Autodesk Inventor part; units mm, degrees
ref_plane "YZ Plane" through (0, 0, 0) normal (1, 0, 0) x (0, 1, 0)
ref_plane "XZ Plane" through (0, 0, 0) normal (0, 1, 0) x (-1, 0, 0)
ref_plane "XY Plane" through (0, 0, 0) normal (0, 0, 1) x (1, 0, 0)
sketch "스케치1" plane through (0, 0, 0) normal (0, 0, 1) x (1, 0, 0)
  line L0 (118.1968, 6) -> (118.1968, 0)
  line L1 (0, 0) -> (2.3, 0)
  line L2 (2.3, 0) -> (2.3, -6)
  line L3 (150, -6) -> (2.3, -6)
  line L4 (150, -6) -> (150, 6)
  line L5 (0, 6) -> (150, 6)
  line L6 (0, 0) -> (0, 6)
  line L7 (150, -6) -> (0, -6)
  line L8 (0, -6) -> (0, 0)
  line L9 (0, 0) -> (150, 0)
  line L10 (150, 0) -> (150, -6)
  line L11 (150, -6) -> (144, -6)
  line L12 (144, -6) -> (144, 0)
  line L13 (144, 0) -> (150, 0)
  line L14 (150, 0) -> (150, -6)
  line L15 (122.25, 6) -> (131.75, 6)
  line L16 (128.025, 6) -> (128.025, 0)
  line L17 (125.975, 6) -> (125.975, 0)
  line L18 (127, 0) -> (127, 6)
  line L19 (104, 0) -> (104, -6)
  line L20 (104, -6) -> (110, -6)
  line L21 (110, -6) -> (110, 0)
  line L22 (110, 0) -> (104, 0)
  line L23 (104, 0) -> (104, -6)
  line L24 (75, -6) -> (75, 6)
  line L25 (0, 0) -> (0, -6)
  line L26 (0, -6) -> (6, -6)
  line L27 (6, 0) -> (0, 0)
  line L28 (0, 0) -> (0, -6)
  line L29 (40, 0) -> (46, 0)
  line L30 (150, -6) -> (144, -6)
  line L31 (144, -6) -> (144, 0)
  line L32 (144, 0) -> (150, 0)
  line L33 (150, 0) -> (150, -6)
  line L34 (110, -6) -> (104, -6)
  line L35 (104, -6) -> (104, 0)
  line L36 (104, 0) -> (110, 0)
  line L37 (110, 0) -> (110, -6)
  line L38 (0, 0) -> (0, -6)
  line L39 (0, -6) -> (6, -6)
  line L40 (6, -6) -> (6, 0)
  line L41 (6, 0) -> (0, 0)
  line L42 (0, 0) -> (0, -6)
  line L43 (40, -6) -> (40, 0)
  line L44 (46, -6) -> (40, -6)
  line L45 (46, 0) -> (46, -6)
  line L46 (46, 0) -> (46, -6)
  line L47 (40, 0) -> (46, 0)
  line L48 (0, -6) -> (6, -6)
  line L49 (6, -6) -> (6, 0)
  line L50 (6, 0) -> (0, 0)
  line L51 (0, 0) -> (0, -6)
  line L52 (40, -6) -> (46, -6)
  line L53 (46, -6) -> (46, 0)
  line L54 (46, 0) -> (40, 0)
  line L55 (40, 0) -> (40, -6)
  line L56 (150, 0) -> (0, 0)
  line L57 (0, 0) -> (0, -125.2)
  line L58 (0, -125.2) -> (150, -125.2)
  line L59 (150, -125.2) -> (150, 0)
  line L60 (150, -62.6) -> (0, -62.6)
  line L61 (0, -125.2) -> (2.3, -125.2)
  line L62 (2.3, -125.2) -> (2.3, -119.2)
  line L63 (150, -119.2) -> (2.3, -119.2)
  line L64 (150, -119.2) -> (0, -119.2)
  line L65 (0, -119.2) -> (0, -125.2)
  line L66 (0, -125.2) -> (150, -125.2)
  line L67 (150, -125.2) -> (150, -119.2)
  line L68 (150, -119.2) -> (144, -119.2)
  line L69 (144, -119.2) -> (144, -125.2)
  line L70 (144, -125.2) -> (150, -125.2)
  line L71 (150, -125.2) -> (150, -119.2)
  line L72 (110, -119.2) -> (110, -125.2)
  line L73 (104, -119.2) -> (110, -119.2)
  line L74 (104, -125.2) -> (104, -119.2)
  line L75 (104, -125.2) -> (104, -119.2)
  line L76 (110, -125.2) -> (104, -125.2)
  line L77 (40, -125.2) -> (46, -125.2)
  line L78 (0, -125.2) -> (0, -119.2)
  line L79 (0, -119.2) -> (6, -119.2)
  line L80 (0, -125.2) -> (0, -119.2)
  line L81 (6, -125.2) -> (0, -125.2)
  line L82 (150, -119.2) -> (144, -119.2)
  line L83 (144, -119.2) -> (144, -125.2)
  line L84 (144, -125.2) -> (150, -125.2)
  line L85 (150, -125.2) -> (150, -119.2)
  line L86 (110, -119.2) -> (104, -119.2)
  line L87 (104, -119.2) -> (104, -125.2)
  line L88 (104, -125.2) -> (110, -125.2)
  line L89 (110, -125.2) -> (110, -119.2)
  line L90 (0, -125.2) -> (0, -119.2)
  line L91 (0, -119.2) -> (6, -119.2)
  line L92 (6, -119.2) -> (6, -125.2)
  line L93 (6, -125.2) -> (0, -125.2)
  line L94 (0, -125.2) -> (0, -119.2)
  line L95 (6, -119.2) -> (6, -125.2)
  line L96 (0, -125.2) -> (0, -119.2)
  line L97 (0, -119.2) -> (6, -119.2)
  line L98 (6, -125.2) -> (0, -125.2)
  line L99 (40, -119.2) -> (40, -125.2)
  line L100 (40, -125.2) -> (40, -119.2)
  line L101 (46, -119.2) -> (40, -119.2)
  line L102 (46, -125.2) -> (46, -119.2)
  line L103 (46, -125.2) -> (46, -119.2)
  line L104 (46, -119.2) -> (46, -125.2)
  line L105 (40, -119.2) -> (46, -119.2)
  line L106 (46, -125.2) -> (40, -125.2)
  line L107 (40, -125.2) -> (46, -125.2)
  line L108 (150, -125.2) -> (0, -125.2)
  point P0 (21.975, 0)
  point P1 (24.025, 0)
  point P2 (31.8032, 0)
  point P3 (21.975, 0)
  point P4 (24.025, 0)
  point P5 (23, 0)
  point P6 (118.1968, -125.2)
  point P7 (128.025, -125.2)
  point P8 (125.975, -125.2)
  point P9 (127, -125.2)
  point P10 (75, -119.2)
  point P11 (24.025, -125.2)
  point P12 (21.975, -125.2)
  point P13 (24.025, -125.2)
  point P14 (23, -125.2)
  point P15 (21.975, -125.2)
  point P16 (31.8032, -125.2)
  dimension "d0" = 125.2
extrude "돌출1" add sketch "스케치1" along normal blind 6 contours L9 L12 L3 L21 | L24 L3 L45 L9 | L9 L19 L3 L24 | L3 L59 L60 L57 L7 | L43 L3 L40 L9 | L60 L59 L63 L64 L57
sketch "스케치2" plane through (0, 0, 0) normal (0, 0, -1) x (-1, 0, 0)
  circle A0 centre (-72.2193, -29.1573) radius 1.55
  circle A1 centre (-75, -39.8) radius 1.5
  circle A2 centre (-75, -39.8) radius 13.9
  circle A3 centre (-75, -39.8) radius 5.2
  circle A4 centre (-75, -39.8) radius 1.6
  point P0 (0, 0)
  dimension "d5" = 0.1
extrude "돌출2" cut sketch "스케치2" against normal up to next contours A1 | A4
sketch "스케치5" plane through (0, 0, 6) normal (0, 0, 1) x (1, 0, 0)
  line L0 (6, 0) -> (6, -6)
  line L1 (6, -6) -> (0, -6)
  line L2 (0, -6) -> (0, -119.2)
  line L3 (150, -119.2) -> (150, -6)
  line L4 (150, -6) -> (144, -6)
  line L5 (144, -6) -> (144, 0)
  line L6 (144, 0) -> (110, 0)
  line L7 (110, 0) -> (110, -6)
  line L8 (110, -6) -> (104, -6)
  line L9 (104, -6) -> (104, 0)
  line L10 (104, 0) -> (46, 0)
  line L11 (46, 0) -> (46, -6)
  line L12 (46, -6) -> (40, -6)
  line L13 (40, -6) -> (40, 0)
  line L14 (40, 0) -> (6, 0)
  circle A0 centre (75, -39.8) radius 1.6
  circle A1 centre (40, -6) radius 1
  circle A2 centre (46, -6) radius 1
  circle A3 centre (40, 0) radius 1
  circle A4 centre (46, 0) radius 1
  circle A5 centre (6, 0) radius 1
  line L15 (6, 0) -> (6, -6)
  circle A6 centre (6, -6) radius 1
  circle A7 centre (0, -6) radius 1
  circle A8 centre (104, -6) radius 1
  circle A9 centre (104, 0) radius 1
  line L16 (110, -6) -> (104, -6)
  circle A10 centre (110, -6) radius 1
  circle A11 centre (110, 0) radius 1
  circle A12 centre (144, -6) radius 1
  line L17 (144, 0) -> (110, 0)
  circle A13 centre (144, 0) radius 1
  circle A14 centre (150, -6) radius 1
  circle A15 centre (123.8, -69.5) radius 1
  circle A16 centre (123.8, -63.1) radius 1
  circle A17 centre (130.2, -69.5) radius 1
  line L18 (130.2, -69.5) -> (130.2, -63.1)
  circle A18 centre (130.2, -63.1) radius 1
  circle A19 centre (19.8, -69.5) radius 1
  circle A20 centre (19.8, -63.1) radius 1
  circle A21 centre (26.2, -69.5) radius 1
  circle A22 centre (26.2, -63.1) radius 1
  line L19 (0, -119.2) -> (150, -119.2)
  point P0 (0, 0)
  point P1 (149, -6)
  point P2 (150, -7)
  point P3 (144, -5)
  point P4 (145, -6)
  point P5 (143, 0)
  point P6 (144, -1)
  dimension "d32" = 2
  dimension "d33" = 2
  dimension "d34" = 2
  dimension "d35" = 2
  dimension "d36" = 2
  dimension "d37" = 2
  dimension "d38" = 2
  dimension "d39" = 2
  dimension "d40" = 2
  dimension "d41" = 2
  dimension "d42" = 2
  dimension "d43" = 2
  dimension "d44" = 2
  dimension "d45" = 2
  dimension "d46" = 2
  dimension "d47" = 2
  dimension "d48" = 2
  dimension "d49" = 2
  dimension "d50" = 2
  dimension "d51" = 2
  dimension "d52" = 2
  dimension "d53" = 2
extrude "돌출5" cut sketch "스케치5" against normal up to next contours L14 A5 L0 | L0 A5 L14 | A6 L1 L0 | L0 L1 A6 | A3 L13 L14 | L14 L13 A3 | A7 L2 L1 | L1 L2 A7 | A1 L12 L13 | L13 L12 A1 | A2 L11 L12 | L12 L11 A2 | A14 L4 L3 | A4 L10 L11 | L11 L10 A4 | A12 L5 L4 | A9 L9 L10 | L10 L9 A9 | A13 L6 L5 | A8 L8 L9 | L9 L8 A8 | A11 L7 L6 | L6 L7 A11 | A10 L7 L8 | L8 L7 A10 picked at (149.7812, -6.6253) picked at (143.8112, -6.634) picked at (143.7812, -0.6253)
sketch "스케치6" plane through (0, 0, 6) normal (0, 0, 1) x (1, 0, 0)
  line L0 (6, -6) -> (6, 0)
  line L1 (0, 0) -> (6, 0)
  line L2 (0, -6) -> (0, 0)
  line L3 (0, -6) -> (6, -6)
  line L4 (40, 0) -> (40, -6)
  line L5 (40, -6) -> (46, -6)
  line L6 (46, -6) -> (46, 0)
  line L7 (40, 0) -> (46, 0)
  line L8 (40, 0) -> (6, 0)
  line L9 (23, 0) -> (23, -6)
  circle A0 centre (23, -3) radius 1.35
  line L10 (104, 0) -> (104, -6)
  line L11 (104, -6) -> (110, -6)
  line L12 (110, -6) -> (110, 0)
  line L13 (104, 0) -> (110, 0)
  line L14 (144, 0) -> (144, -6)
  line L15 (144, -6) -> (150, -6)
  line L16 (150, -6) -> (150, 0)
  line L17 (144, 0) -> (150, 0)
  line L18 (104, -3) -> (46, -3)
  line L19 (75, -3) -> (75, 0)
  line L20 (103, 0) -> (47, 0)
  line L21 (75, -3) -> (104, -3)
  line L22 (89.5, -3) -> (89.5, 0)
  line L23 (75, -3) -> (46, -3)
  line L24 (60.5, -3) -> (60.5, 0)
  circle A1 centre (89.5, -3) radius 1.3
  circle A2 centre (60.5, -3) radius 1.3
  circle A3 centre (127, -3) radius 1.35
  point P0 (127, -6)
  dimension "d58" = 2.6
  dimension "d59" = 2.6
extrude "돌출6" cut sketch "스케치6" against normal up to next contours A2 L24 L18 | L18 A2 | A0 L9 | L9 A0 | L24 A2 L18 | A1 L22 L18 | L18 A1 | L22 A1 L18 | A3
sketch "스케치13" plane through (0, 0, 6) normal (0, 0, 1) x (1, 0, 0)
  circle A0 centre (82.7782, -32.0218) radius 1.55
  circle A1 centre (82.7782, -32.0218) radius 1.55
  circle A2 centre (75, -28.8) radius 1.55
  circle A3 centre (75, -39.8) radius 1.6
  circle A4 centre (82.7782, -32.0218) radius 1.55
  circle A5 centre (75, -28.8) radius 1.55
  circle A6 centre (67.2218, -32.0218) radius 1.55
  circle A7 centre (64, -39.8) radius 1.55
  circle A8 centre (67.2218, -47.5782) radius 1.55
  circle A9 centre (75, -50.8) radius 1.55
  circle A10 centre (82.7782, -47.5782) radius 1.55
  circle A11 centre (86, -39.8) radius 1.55
  point P0 (0, 0)
  dimension "d77" = 360
extrude "돌출9" cut sketch "스케치13" against normal blind 10 contours A0 | A2 | A6 | A7 | A8 | A9 | A10 | A11
properties part number "부품49" material "PMMA 플라스틱"
CAD build for the part. Positions are in the model's coordinates, mm. A direction names the side the tool comes from. Round coordinates to 2 decimals unless told otherwise and drop trailing zeros. Order: outer loops, then holes, each group sorted by start corner. A loop starts at its lowest first (then second) coordinate and runs counter-clockwise, first axis right, second up. Notation, with made-up numbers: (17.5, 0) -> (68.5, 0) arc R29 cw to (68.5, 38) -> close; hole circle Ø2 at (52.5, -1.75). An arc over 180 degrees is marked (long way). Write each question's results on one line, items separated by ' | '.
1. Pull direction Y, two halves, no side cores. Call faces 1 (the face through (76.478, -28.334, 3.042)), 2 (the face through (74, -59, 0)), 3 (the face through (43, -6, 3)): pulls with the +Y half, pulls with the -Y half, needs draft (parallel to the pull), parting line crosses it, or undercut.
Findings below:
face 1: undercut | face 2: needs draft | face 3: pulls with the +Y half
2. Cut at A-A (y = -50.8). Give the cut face in (x, z).
Findings below:
outline: (0, 0) -> (73.45, 0) -> (73.45, 6) -> (0, 6) -> close; (76.55, 0) -> (150, 0) -> (150, 6) -> (76.55, 6) -> close
3. 3-axis set-ups, long thin cutter, end or side, ignore diameter. For faces 4 (the face through (107, -6, 3)), 5 (the face through (147, -6, 3)), 6 (the face through (23, 0, 3)): which of +Z, -Z, +X, -X, +Y, -Y reach the whole face in a straight line?
Findings below:
face 4: +Z, -Z, +Y | face 5: +Z, -Z, +X, +Y | face 6: +Z, -Z, +X, -X, +Y
4. Wall check: line 1 along Y through (x, z) = (60.5, 4.15); line 2 along Y through (x, z) = (68, 4.4); line 3 along Y through (x, z) = (63, 0.5). Give the ranges that are in metal, low to high. Write a range as [from, to].
Findings below:
line 1: y = [-119.2, -4.3], [-1.7, 0] | line 2: y = [-119.2, -48.92], [-46.24, -33.36], [-30.68, 0] | line 3: y = [-119.2, -40.98], [-38.62, 0]
5. Flat gauge pins, fed straight in: P1, Ø2, axis at y = -3, z = 2.5, coming from the -X side; P2, Ø1.2, axis at x = 148, z = 3.5, coming from the +Y side; P3, Ø2, axis at y = -2.5, z = 1.5, coming from the +X side. Where does each tip first touch, or does it go through?
Findings below:
P1: stops at x = 6 | P2: stops at y = -6 | P3: stops at x = 144
6. Cut at B-B (x = 75). Give the cut face in (y, z).
Findings below:
outline: (-119.2, 0) -> (-52.35, 0) -> (-52.35, 6) -> (-119.2, 6) -> close; (-49.25, 0) -> (-41.4, 0) -> (-41.4, 6) -> (-49.25, 6) -> close; (-38.2, 0) -> (-30.35, 0) -> (-30.35, 6) -> (-38.2, 6) -> close; (-27.25, 0) -> (0, 0) -> (0, 6) -> (-27.25, 6) -> close
